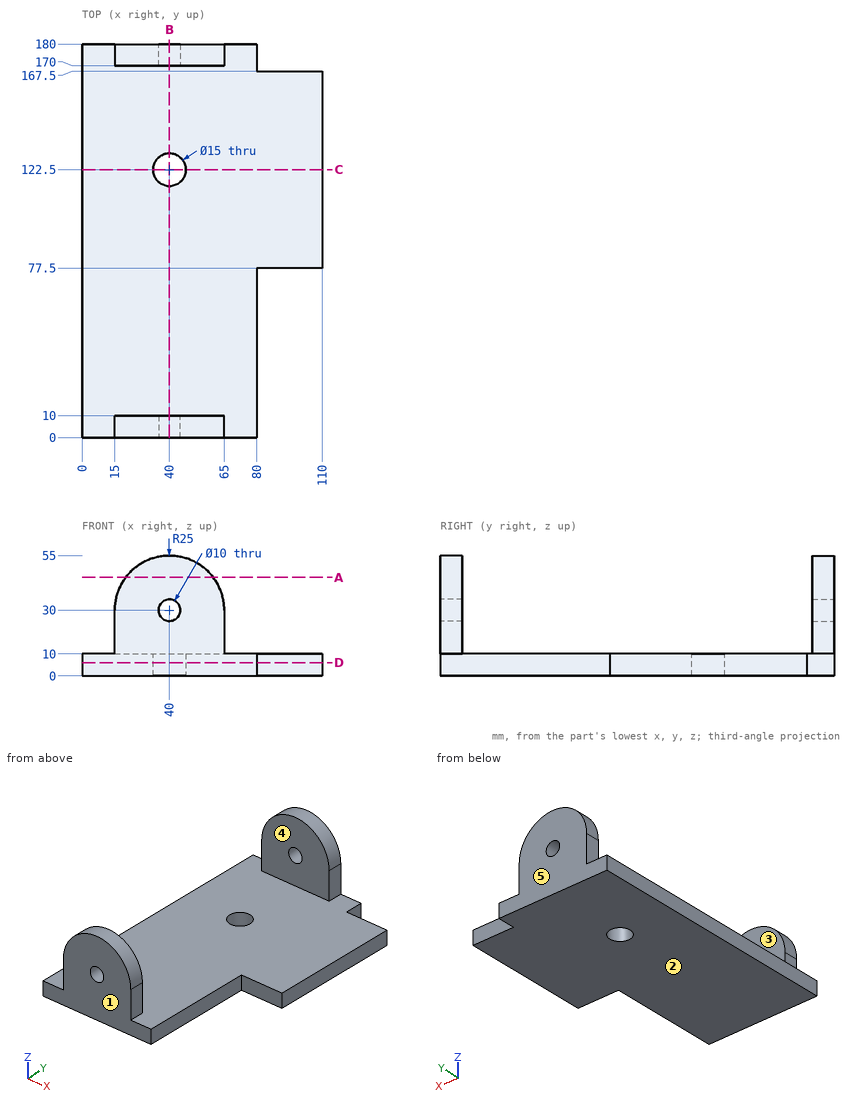
Design review of the part shown in the three views and the two pictorial views. Dimensions are in mm from the part's minimum x, y and z. A direction names the side the tool comes from. Round coordinates to 2 decimals unless told otherwise and drop trailing zeros. Loops run counter-clockwise (first coordinate to the right, second up) from the corner with the lowest first, then second, coordinate; pieces in that order, holes last.
Q1. Add section D-D on z = 6. Write out the cut boundary in (x, y), plus the area to 3 significant figures.
Result sheet:
outline: (0, 0) - (80, 0) - (80, 77.5) - (110, 77.5) - (110, 167.5) - (80, 167.5) - (80, 180) - (0, 180) - close; hole circle Ø15 at (40, 122.5)
area: 16,900 mm2
Q2. Mouldability with a two-part tool opening along Y and no side actions: class the marked faces 1, 2 and 3 as +Y half, -Y half, draft (parallel to the pull), parting line (faces both ways), or undercut.
Result sheet:
face 1: -Y half
face 2: draft
face 3: undercut
Q3. Insertion check: pin 1 Ø11 at (y, z) = (174, 24) entering from +X; pin 2 Ø11 at (y, z) = (172.5, 16) entering from -X; pin 3 Ø8 at (x, z) = (40, 30) entering from +Y; pin 4 Ø3 at (x, z) = (93, 5) entering from +Y. Each pin has a flat end and moves straight along its axis. Give the tip position at first contact, or say it passes through.
Result sheet:
pin 1: stops at x = 65
pin 2: stops at x = 15
pin 3: passes through
pin 4: stops at y = 167.5
Q4. Add section C-C on y = 122.5. Write out the cut boundary in (x, z).
Result sheet:
outline: (0, 0) - (32.5, 0) - (32.5, 10) - (0, 10) - close; (47.5, 0) - (110, 0) - (110, 10) - (47.5, 10) - close
Q5. To check wall thickness, follow line 1 along X through (y, z) = (122.5, 7.75); line 2 along X through (y, z) = (173, 30); line 3 along Y through (x, z) = (48, 21.5). State the ranges of each line that lie inside material, in increasing order.
Result sheet:
line 1: x = 0 to 32.5, 47.5 to 110
line 2: x = 15 to 35, 45 to 65
line 3: y = 0 to 10, 170 to 180
Q6. Add section A-A on z = 45. Write out the cut boundary in (x, y).
Result sheet:
outline: (20, 0) - (60, 0) - (60, 10) - (20, 10) - close; (20, 170) - (60, 170) - (60, 180) - (20, 180) - close
Q7. Add section B-B on x = 40. Write out the cut boundary in (y, z), plus the area to 3 significant figures.
Result sheet:
outline: (0, 0) - (115, 0) - (115, 10) - (10, 10) - (10, 25) - (0, 25) - close; (0, 35) - (10, 35) - (10, 55) - (0, 55) - close; (130, 0) - (180, 0) - (180, 25) - (170, 25) - (170, 10) - (130, 10) - close; (170, 35) - (180, 35) - (180, 55) - (170, 55) - close
area: 2,350 mm2
Q8. Machinability: for the marked faces 4 and 5, which of the approach directions +Z, -Z, +X, -X, +Y, -Y give a long, thin tool a straight path to every point of the face, cutting with its end or side? Answer none if there is none.
Result sheet:
face 4: +Z, +X, -X
face 5: +Z, -Z, +X, -X, +Y
